Can you work these out from the model? Positions are in its coordinate system, mm. Face numbers are marked on the shaded views. A direction names the side the tool comes from. Give positions to 0.01 mm unless a question says otherwise; leave off trailing zeros. Write each loop counter-clockwise with the first axis right and the second up, starting at its lowest first coordinate (ties: lowest second). Pieces come first, ordered by that corner, then holes.
from build123d import *

# Parameters (mm, degrees)
EXTRUDE_1_DEPTH     = 25
SKETCH_2_R          = 2.55
CUT_EXTRUDE_1_DEPTH = 5
FILLET_1_R          = 2
FILLET_2_R          = 0.5
SKETCH_3_R          = 2.55
CUT_EXTRUDE_2_DEPTH = 35


with BuildPart() as part:
    # 草图1 → 凸台-拉伸1 (new body)
    with BuildSketch(Plane.XY):
        Polygon((0, 0), (23.51262021, 0), (23.51262021, 3), (0, 3), (-4, 3), (-4, -19), (0, -19), (23.51262021, -19), (23.51262021, -16), (0, -16), align=None)
    extrude(amount=EXTRUDE_1_DEPTH)

    # 草图2 → 切除-拉伸1 (cut)
    with BuildSketch(Plane.ZY.offset(4)):
        with Locations(Location((12.5, -8, 0), (0, 0, 270))):
            Circle(SKETCH_2_R)
    extrude(amount=-CUT_EXTRUDE_1_DEPTH, mode=Mode.SUBTRACT)

    # 圆角1
    fillet_1_edges = [part.edges().sort_by_distance(p)[0] for p in [
        (0, -16, 12.5),
        (-4, -19, 12.5),
        (-4, 3, 12.5),
        (0, 0, 12.5),
    ]]
    fillet(fillet_1_edges, radius=FILLET_1_R)

    # 圆角2
    fillet_2_edges = [part.edges().sort_by_distance(p)[0] for p in [
        (23.51262021, -16, 12.5),
        (23.51262021, -19, 12.5),
        (23.51262021, 3, 12.5),
        (23.51262021, 0, 12.5),
    ]]
    fillet(fillet_2_edges, radius=FILLET_2_R)

    # 草图3 → 切除-拉伸2 (cut)
    with BuildSketch(Plane(origin=(0, 3, 0), x_dir=(1, 0, 0), z_dir=(0, 1, 0))):
        with Locations(Location((13, -12.5, 0), (0, 0, 270))):
            Circle(SKETCH_3_R)
    extrude(amount=-CUT_EXTRUDE_2_DEPTH, mode=Mode.SUBTRACT)


solid = part.part
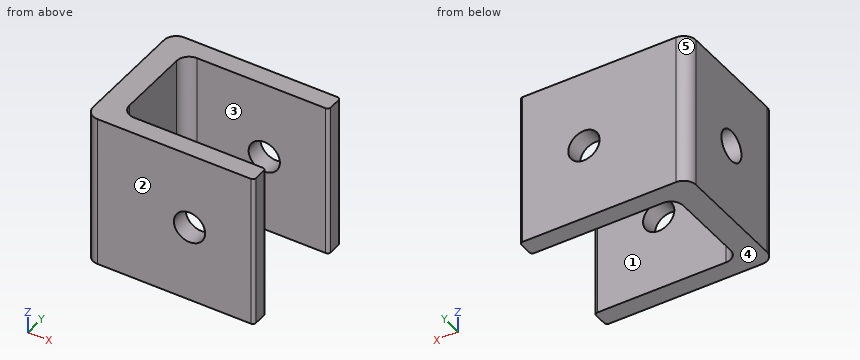
(1) Imagine slicing it at C-C, the plane z = 12.5. Write out the boundary of the cut face in (x, y).
Returned:
outline: (-4, -17) arc R2 ccw to (-2, -19) - (10.45, -19) - (10.45, -16) - (2, -16) arc R2 cw to (0, -14) - (0, -10.55) - (-4, -10.55) - close; (-4, -5.45) - (0, -5.45) - (0, -2) arc R2 cw to (2, 0) - (10.45, 0) - (10.45, 3) - (-2, 3) arc R2 ccw to (-4, 1) - close; (15.55, -19) - (23.01, -19) arc R0.5 ccw to (23.51, -18.5) - (23.51, -16.5) arc R0.5 ccw to (23.01, -16) - (15.55, -16) - close; (15.55, 0) - (23.01, 0) arc R0.5 ccw to (23.51, 0.5) - (23.51, 2.5) arc R0.5 ccw to (23.01, 3) - (15.55, 3) - close
(2) If we mould it in two halves opening along Y, with no side actions, what happens to the marked faces 3, 4 and 5? For each: +Y half, -Y half, draft (parallel to the pull), parting line (faces both ways), or undercut.
Returned:
face 3: undercut
face 4: draft
face 5: +Y half
(3) Imagine slicing it at D-D, the plane x = 20.5. Write out the boundary of the cut face in (y, z), plus the area to 3 significant figures.
Returned:
outline: (-19, 0) - (-16, 0) - (-16, 25) - (-19, 25) - close; (0, 0) - (3, 0) - (3, 25) - (0, 25) - close
area: 150 mm2
(4) If I drill on L1, parallel to Y at x = 2.25, z = 11.75; L2, parallel to Z at x = -2.25, y = -8; L3, parallel to X at y = -18, z = 12.5, over which ranges is the centre line in solid material (lowest first)?
Returned:
L1: y = -19 to -16, 0 to 3
L2: z = 0 to 9.95, 15.05 to 25
L3: x = -3.73 to 10.45, 15.55 to 23.51
(5) For the marked faces 1 and 2, which set-ups out of +Z, -Z, +X, -X, +Y, -Y let a thin tool reach every point of the face, with its end or its side?
Returned:
face 1: +Z, -Z, +X
face 2: +Z, -Z, +X, -X, -Y
(6) Imagine slicing it at B-B, the plane y = -8. Write out the boundary of the cut face in (x, z), plus the area to 3 significant figures.
Returned:
outline: (-4, 0) - (0, 0) - (0, 9.95) - (-4, 9.95) - close; (-4, 15.05) - (0, 15.05) - (0, 25) - (-4, 25) - close
area: 79.6 mm2
(7) Imagine slicing it at A-A, the plane x = 13. Write out the boundary of the cut face in (y, z).
Returned:
outline: (-19, 0) - (-16, 0) - (-16, 9.95) - (-19, 9.95) - close; (-19, 15.05) - (-16, 15.05) - (-16, 25) - (-19, 25) - close; (0, 0) - (3, 0) - (3, 9.95) - (0, 9.95) - close; (0, 15.05) - (3, 15.05) - (3, 25) - (0, 25) - close
(8) Will these pins go through, and if not, where does the flat tip stop? P1, Ø1.5, axis at y = -10, z = 4, coming from the +X side; P2, Ø3, axis at x = 13, z = 12.5, coming from the +Y side.
Returned:
P1: stops at x = 0
P2: passes through
